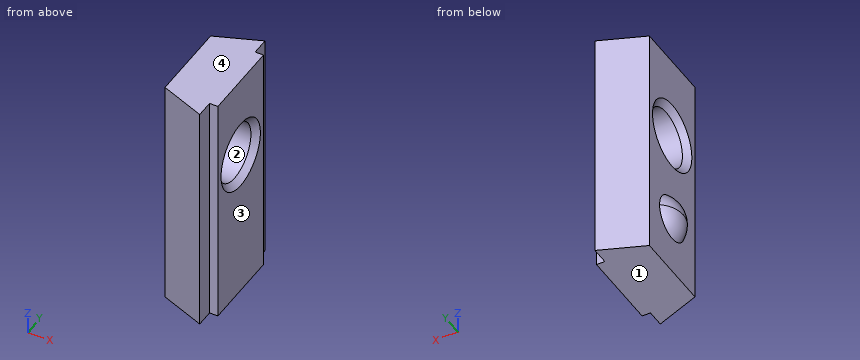
```python
from build123d import *
from build123d.topology import SkipClean

# Parameters (mm, degrees)
EXTRUDE_1_DEPTH      = 8.5
EXTRUDE_1_DEPTH_BACK = 8.5


with BuildPart() as part:
    # Sketch 1 → Extrude 1 (new, two sides)
    with BuildSketch(Plane.XY) as extrude_1_sk:
        Polygon((0, -2.9), (3.2, -4.15), (3.2, -2.9), (3.8, -2.9), (3.8, 2.9), (3.2, 2.9), (3.2, 4.15), (0, 2.9), align=None)
    extrude(amount=EXTRUDE_1_DEPTH)
    extrude(extrude_1_sk.sketch, amount=-EXTRUDE_1_DEPTH_BACK)

    # Sketch 2 → Cut-Revolve 1 (revolve, cut)
    with BuildSketch(Plane.XY.offset(2.5), mode=Mode.PRIVATE) as cut_revolve_1_sk:
        Polygon((0, 0), (0, 2.5), (0.433, 2.067), (3.367, 2.067), (3.8, 2.5), (3.8, 0), align=None)
    revolve(cut_revolve_1_sk.sketch.rotate(Axis((3.8, 0, 2.5), (-1, 0, 0)), 270), axis=Axis((3.8, 0, 2.5), (-1, 0, 0)), mode=Mode.SUBTRACT)

    # Sketch 3 → Revolve 1 (revolve)
    with SkipClean():  # the faces are left unmerged after this step: merging them gives an invalid solid
        with BuildSketch(Plane.XY.offset(-4.25)):
            with BuildLine():
                Line((1.2, 2), (1.2, -2))
                ThreePointArc((1.2, -2), (-0.8, 0), (1.2, 2))
            make_face()
        revolve(axis=Axis((1.2, 3.2, -4.25), (0, -1, 0)))


solid = part.part
```
The model under review builds one solid part; all positions refer to its coordinate system, in mm. Face numbers are marked on the shaded views. Give positions to 0.01 mm unless a question says otherwise; leave off trailing zeros. Loops run counter-clockwise (first coordinate to the right, second up) from the corner with the lowest first, then second, coordinate; pieces in that order, holes last. Notation, with made-up numbers: (78, -22.5) - (87, -22.5) arc R31 ccw to (87, 15.5) - close; hole circle Ø5 at (38.25, 28). An arc over 180 degrees is marked (long way). Answer as a JSON object with one key per item and string values.
Q1. Add section D-D on x = 1.05. State the section outline as (y, z) points, plus the area to 3 significant figures.
Worked out:
{"outline": "(-3.31, -8.5) - (3.31, -8.5) - (3.31, 8.5) - (-3.31, 8.5) - close; hole circle Ø4.13 at (0, 2.5)", "area": "99.1 mm^2"}
Q2. To check wall thickness, follow line 1 along Y through (x, z) = (3.45, 8); line 2 along X through (y, z) = (2.75, -5.5); line 3 along Y through (x, z) = (1.05, 2.5). State the ranges of each line that lie inside material, in increasing order.
Worked out:
{"line 1": "y = -2.9 to 2.9", "line 2": "x = 0 to 3.8", "line 3": "y = -3.31 to -2.07, 2.07 to 3.31"}
Q3. Add section A-A on z = 2.5. State the section outline as (x, y) points.
Worked out:
{"outline": "(0, -2.9) - (3.2, -4.15) - (3.2, -2.9) - (3.8, -2.9) - (3.8, -2.5) - (3.37, -2.07) - (0.43, -2.07) - (0, -2.5) - close; (0, 2.5) - (0.43, 2.07) - (3.37, 2.07) - (3.8, 2.5) - (3.8, 2.9) - (3.2, 2.9) - (3.2, 4.15) - (0, 2.9) - close"}
Q4. Mouldability with a two-part tool opening along Z and no side actions: class the marked faces 1, 2, 3 and 4 as +Z half, -Z half, draft (parallel to the pull), parting line (faces both ways), or undercut.
Worked out:
{"face 1": "-Z half", "face 2": "undercut", "face 3": "draft", "face 4": "+Z half"}
Q5. Insertion check: pin 1 (1.5 mm diameter, centred on y = 1, z = -4.5, fed in from -X); pin 2 (1 mm diameter, centred on x = 2, z = 4, fed in from -Y); pin 3 (0.5 mm diameter, centred on x = 3.5, z = -3, fed in from -Y); pin 4 (1.4 mm diameter, centred on y = -3, z = 4, fed in from +X). Each pin has a flat end and moves straight along its axis. Give the tip position at first contact, or say it passes through.
Worked out:
{"pin 1": "stops at x = -0.78", "pin 2": "stops at y = -3.88", "pin 3": "stops at y = -2.9", "pin 4": "stops at x = 3.8"}
Q6. Add section B-B on x = 3.55. State the section outline as (y, z) points.
Worked out:
{"outline": "(-2.9, -8.5) - (2.9, -8.5) - (2.9, 8.5) - (-2.9, 8.5) - close; hole circle Ø4.5 at (0, 2.5)"}
Q7. Add section C-C on z = 6. State the section outline as (x, y) points.
Worked out:
{"outline": "(0, -2.9) - (3.2, -4.15) - (3.2, -2.9) - (3.8, -2.9) - (3.8, 2.9) - (3.2, 2.9) - (3.2, 4.15) - (0, 2.9) - close"}
